Verification items for the finished model (mm, model axes). Face numbers are marked on the shaded views. A direction names the side the tool comes from. Coordinates: 2 decimals unless noted, no trailing zeros. Order: outer loops, then holes, each group sorted by start corner. A loop starts at its lowest first (then second) coordinate and runs counter-clockwise, first axis right, second up.
Q1. Cross-section at B-B, the plane x = 10. Record the boundary of the cut face in (y, z).
Q2. Cross-section at A-A, the plane y = 70. Record the boundary of the cut face in (x, z).
Q3. Depth check by flat-ended pin: P1, Ø12, axis at y = 13, z = 11, coming from the -X side; P2, Ø1, axis at x = -1, y = 64, coming from the -Z side; P3, Ø8, axis at y = 57, z = 16.5, coming from the -X side; P4, Ø4, axis at x = 33.5, z = 10, coming from the +Y side. Enter the tip coordinate at first touch or a pass-through.
Q4. Thickness scan on line 1 (Y direction, x = 10, z = 2.5); line 2 (X direction, y = 10, z = 2); line 3 (Z direction, x = -8, y = 45). Record the ranges inside material, lowest first.
Q5. Set-up check for the marked faces 1, 2, 3 and 4: record each of +Z, -Z, +X, -X, +Y, -Y from which the full face is reachable in a straight line by a thin tool's end or side.
Q6. Draft check along Y on the marked faces 5, 6 and 7. Enter one of: pulls with the +Y half, pulls with the -Y half, needs draft (parallel to the pull), parting line crosses it, or undercut.
from build123d import *

# Parameters (mm, degrees)
SKIZZE1_W                       = 20
SKIZZE1_H                       = 80
SKIZZE1_R                       = 4.3
AUFSATZ_LINEAR_AUSTRAGEN1_DEPTH = 7
AUFSATZ_LINEAR_AUSTRAGEN2_DEPTH = 15
SCHNITT_LINEAR_AUSTRAGEN1_DEPTH = 10
F_6_0_6_DURCHMESSER_BOHRUNG1_D  = 6


with BuildPart() as part:
    # Skizze1 → Aufsatz-Linear austragen1 (new body)
    with BuildSketch(Plane.XY):
        with Locations((10, 40)):
            Rectangle(SKIZZE1_W, SKIZZE1_H)
        with Locations((10, 70)):
            Circle(SKIZZE1_R, mode=Mode.SUBTRACT)
        with Locations(Location((10, 10, 0), (0, 0, 180))):  # turned: the seam where the file's is
            Circle(SKIZZE1_R, mode=Mode.SUBTRACT)
    extrude(amount=AUFSATZ_LINEAR_AUSTRAGEN1_DEPTH)

    # Skizze2 → Aufsatz-Linear austragen2 (add)
    with BuildSketch(Plane.XY.offset(7)):
        Polygon((32.882510841, 20.376208379), (20, 29.396639581), (20, 20.79017873), (28.838796965, 14.601186467), align=None)
        Polygon((36.266611816, 25.20920544), (20, 36.599209655), (20, 29.396639581), (32.882510841, 20.376208379), align=None)
        Polygon((40.310325692, 30.984227352), (20, 45.205670506), (20, 36.599209655), (36.266611816, 25.20920544), align=None)
        Polygon((20, 45.205670506), (0, 59.20982127), (0, 50.603360419), (20, 36.599209655), align=None)
        Polygon((20, 36.599209655), (0, 50.603360419), (0, 43.400790345), (20, 29.396639581), align=None)
        Polygon((20, 29.396639581), (0, 43.400790345), (0, 34.794329494), (20, 20.79017873), align=None)
        Polygon((0, 43.400790345), (-16.266611816, 54.79079456), (-20.310325692, 49.015772648), (0, 34.794329494), align=None)
        Polygon((0, 50.603360419), (-12.882510841, 59.623791621), (-16.266611816, 54.79079456), (0, 43.400790345), align=None)
        Polygon((0, 59.20982127), (-8.838796965, 65.398813533), (-12.882510841, 59.623791621), (0, 50.603360419), align=None)
    extrude(amount=AUFSATZ_LINEAR_AUSTRAGEN2_DEPTH)

    # Skizze3 → Schnitt-Linear austragen1 (cut)
    with BuildSketch(Plane.XY.offset(22)):
        Polygon((-16.266611816, 54.79079456), (32.882510841, 20.376208379), (36.266611816, 25.20920544), (-12.882510841, 59.623791621), align=None)
    extrude(amount=-SCHNITT_LINEAR_AUSTRAGEN1_DEPTH, mode=Mode.SUBTRACT)

    # Ø6.0 (6) Durchmesser Bohrung1 (through all)
    with Locations(Plane(origin=(27.819516063, 39.730386413, 0), x_dir=(0.819152044, -0.573576436, 0), z_dir=(0.573576436, 0.819152044, 0))):
        with Locations((2.248462989, -17), (-31.751537011, -17)):
            Hole(F_6_0_6_DURCHMESSER_BOHRUNG1_D / 2)


solid = part.part
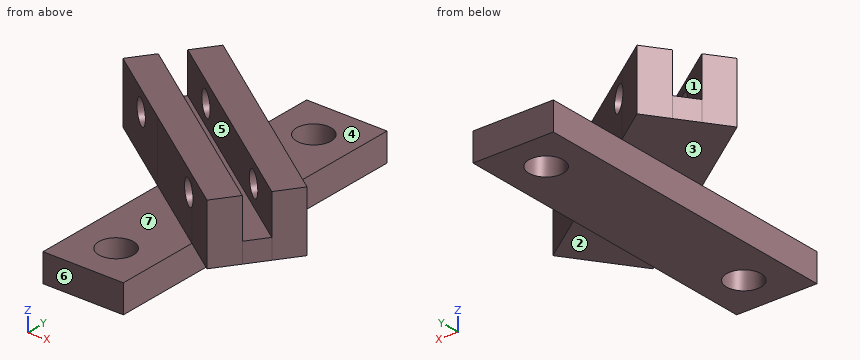
Check values:
1. outline: (0, 0) - (5.7, 0) - (5.7, 7) - (0, 7) - close; (14.3, 0) - (65.7, 0) - (65.7, 7) - (52.21, 7) - (52.21, 22) - (43.6, 22) - (43.6, 12) - (36.4, 12) - (36.4, 22) - (27.79, 22) - (27.79, 7) - (14.3, 7) - close; (74.3, 0) - (80, 0) - (80, 7) - (74.3, 7) - close
2. outline: (0, 0) - (5.7, 0) - (5.7, 7) - (0, 7) - close; (14.3, 0) - (20, 0) - (20, 7) - (14.3, 7) - close
3. P1: stops at x = 0
3. P2: passes through
3. P3: stops at x = -17.52
3. P4: stops at y = 37.15
4. line 1: y = 0 to 5.7, 14.3 to 65.7, 74.3 to 80
4. line 2: x = 0 to 5.7, 14.3 to 20
4. line 3: z = 7 to 14.06, 19.94 to 22
5. face 1: +Z
5. face 2: -Z, +X, +Y, -Y
5. face 3: -Z, -X, +Y, -Y
5. face 4: +Z, +X, +Y
6. face 5: undercut
6. face 6: pulls with the -Y half
6. face 7: needs draft
